```python
from build123d import *

# Parameters (mm, degrees)
SKETCH1_R           = 25
SKETCH1_R_2         = 5.1
SKETCH1_R_3         = 2.5
SKETCH1_W           = 36
SKETCH1_H           = 36
SKETCH1_W_2         = 6
SKETCH1_H_2         = 20
BOSS_EXTRUDE1_DEPTH = 3
BOSS_EXTRUDE2_DEPTH = 43
SKETCH4_W           = 11
SKETCH4_H           = 11
SKETCH4_W_2         = 7
SKETCH4_H_2         = 7
BOSS_EXTRUDE3_DEPTH = 5
SKETCH5_R           = 1.75
CUT_EXTRUDE1_DEPTH  = 5
SKETCH6_R           = 3.5
CUT_EXTRUDE2_DEPTH  = 3


with BuildPart() as part:
    # Sketch1 → Boss-Extrude1 (new body)
    with BuildSketch(Plane(origin=(0, 0, 0), x_dir=(1, 0, 0), z_dir=(0, 1, 0))):
        with BuildLine():
            Line((-20.833630945, -24.478740106), (119.166369055, -24.478740106))
            ThreePointArc((119.166369055, -24.478740106), (122.701902961, -23.014274012), (124.166369055, -19.478740106))
            Line((124.166369055, -19.478740106), (124.166369055, 72.136095087))
            ThreePointArc((124.166369055, 72.136095087), (123.306705208, 74.939239133), (121.023322437, 76.778478541))
            Line((121.023322437, 76.778478541), (75.060410419, 95.163643348))
            ThreePointArc((75.060410419, 95.163643348), (74.148994643, 95.431041828), (73.203457037, 95.521259894))
            Line((73.203457037, 95.521259894), (25.129281073, 95.521259894))
            ThreePointArc((25.129281073, 95.521259894), (24.183743467, 95.431041828), (23.272327691, 95.163643348))
            Line((23.272327691, 95.163643348), (-22.690584327, 76.778478541))
            ThreePointArc((-22.690584327, 76.778478541), (-24.973967097, 74.939239133), (-25.833630945, 72.136095087))
            Line((-25.833630945, 72.136095087), (-25.833630945, -19.478740106))
            ThreePointArc((-25.833630945, -19.478740106), (-24.369164851, -23.014274012), (-20.833630945, -24.478740106))
        make_face()
        with Locations((4.016369055, 8.771259894)):
            Circle(SKETCH1_R, mode=Mode.SUBTRACT)
        with Locations((94.316369055, 8.771259894)):
            Circle(SKETCH1_R, mode=Mode.SUBTRACT)
        with Locations((4.016369055, 67.521259894)):
            Circle(SKETCH1_R_2, mode=Mode.SUBTRACT)
        with Locations((94.316369055, 67.521259894)):
            Circle(SKETCH1_R_2, mode=Mode.SUBTRACT)
        with Locations((19.166369055, 79.316074422)):
            Circle(SKETCH1_R_3, mode=Mode.SUBTRACT)
        with Locations((19.166369055, 59.316074422)):
            Circle(SKETCH1_R_3, mode=Mode.SUBTRACT)
        with Locations((79.166369055, 59.316074422)):
            Circle(SKETCH1_R_3, mode=Mode.SUBTRACT)
        with Locations((79.166369055, 79.316074422)):
            Circle(SKETCH1_R_3, mode=Mode.SUBTRACT)
        with Locations((49.166369055, 67.521259894)):
            Rectangle(SKETCH1_W, SKETCH1_H, mode=Mode.SUBTRACT)
        with Locations((49.166369055, 8.771259894)):
            Rectangle(SKETCH1_W_2, SKETCH1_H_2, mode=Mode.SUBTRACT)
    extrude(amount=BOSS_EXTRUDE1_DEPTH)

    # Sketch2 → Boss-Extrude2 (add)
    with BuildSketch(Plane.XZ):
        with BuildLine():
            Line((-25.833630945, 19.478740106), (-25.833630945, -72.136095087))
            ThreePointArc((-25.833630945, -72.136095087), (-24.973967097, -74.939239133), (-22.690584327, -76.778478541))
            Line((-22.690584327, -76.778478541), (23.272327691, -95.163643348))
            ThreePointArc((23.272327691, -95.163643348), (24.183743467, -95.431041828), (25.129281073, -95.521259894))
            Line((25.129281073, -95.521259894), (73.203457037, -95.521259894))
            ThreePointArc((73.203457037, -95.521259894), (74.148994643, -95.431041828), (75.060410419, -95.163643348))
            Line((75.060410419, -95.163643348), (121.023322437, -76.778478541))
            ThreePointArc((121.023322437, -76.778478541), (123.306705208, -74.939239133), (124.166369055, -72.136095087))
            Line((124.166369055, -72.136095087), (124.166369055, 19.478740106))
            ThreePointArc((124.166369055, 19.478740106), (122.701902961, 23.014274012), (119.166369055, 24.478740106))
            Line((119.166369055, 24.478740106), (-20.833630945, 24.478740106))
            ThreePointArc((-20.833630945, 24.478740106), (-24.369164851, 23.014274012), (-25.833630945, 19.478740106))
        make_face()
        with BuildLine():
            Line((119.166369055, 21.478740106), (-20.833630945, 21.478740106))
            ThreePointArc((-20.833630945, 21.478740106), (-22.247844507, 20.892953668), (-22.833630945, 19.478740106))
            Line((-22.833630945, 19.478740106), (-22.833630945, -72.136095087))
            ThreePointArc((-22.833630945, -72.136095087), (-22.489765406, -73.257352705), (-21.576412297, -73.993048469))
            Line((-21.576412297, -73.993048469), (24.38649972, -92.378213276))
            ThreePointArc((24.38649972, -92.378213276), (24.751066031, -92.485172667), (25.129281073, -92.521259894))
            Line((25.129281073, -92.521259894), (73.203457037, -92.521259894))
            ThreePointArc((73.203457037, -92.521259894), (73.58167208, -92.485172667), (73.94623839, -92.378213276))
            Line((73.94623839, -92.378213276), (119.909150408, -73.993048469))
            ThreePointArc((119.909150408, -73.993048469), (120.822503516, -73.257352705), (121.166369055, -72.136095087))
            Line((121.166369055, -72.136095087), (121.166369055, 19.478740106))
            ThreePointArc((121.166369055, 19.478740106), (120.580582618, 20.892953668), (119.166369055, 21.478740106))
        make_face(mode=Mode.SUBTRACT)
    extrude(amount=BOSS_EXTRUDE2_DEPTH)

    # Sketch4 → Boss-Extrude3 (add)
    with BuildSketch(Plane.XZ):
        with Locations((79.166369055, -79.316074422)):
            Rectangle(SKETCH4_W, SKETCH4_H)
        with Locations((79.166369055, -79.316074422)):
            Rectangle(SKETCH4_W_2, SKETCH4_H_2, mode=Mode.SUBTRACT)
        with Locations((79.166369055, -59.316074422)):
            Rectangle(SKETCH4_W, SKETCH4_H)
        with Locations((79.166369055, -59.316074422)):
            Rectangle(SKETCH4_W_2, SKETCH4_H_2, mode=Mode.SUBTRACT)
        with Locations((19.166369055, -59.316074422)):
            Rectangle(SKETCH4_W, SKETCH4_H)
        with Locations((19.166369055, -59.316074422)):
            Rectangle(SKETCH4_W_2, SKETCH4_H_2, mode=Mode.SUBTRACT)
        with Locations((19.166369055, -79.316074422)):
            Rectangle(SKETCH4_W, SKETCH4_H)
        with Locations((19.166369055, -79.316074422)):
            Rectangle(SKETCH4_W_2, SKETCH4_H_2, mode=Mode.SUBTRACT)
    extrude(amount=BOSS_EXTRUDE3_DEPTH)

    # Sketch5 → Cut-Extrude1 (cut)
    with BuildSketch(Plane.XZ):
        with Locations((-17.833630945, 16.478740106)):
            Circle(SKETCH5_R)
        with Locations((116.166369055, 16.478740106)):
            Circle(SKETCH5_R)
        with Locations((-17.833630945, -63.521259894)):
            Circle(SKETCH5_R)
        with Locations((116.166369055, -63.521259894)):
            Circle(SKETCH5_R)
    extrude(amount=-CUT_EXTRUDE1_DEPTH, mode=Mode.SUBTRACT)

    # Sketch6 → Cut-Extrude2 (cut)
    with BuildSketch(Plane(origin=(0, 0, -95.521259894), x_dir=(-1, 0, 0), z_dir=(0, 0, -1))):
        with Locations((-49.166369055, -29.5)):
            Circle(SKETCH6_R)
    extrude(amount=-CUT_EXTRUDE2_DEPTH, mode=Mode.SUBTRACT)


solid = part.part
```
Check sheet for the modelled part. Datum: model origin and axes. Units: mm. A direction names the side the tool comes from. Coordinates: 2 decimals unless noted, no trailing zeros. Order: outer loops, then holes, each group sorted by start corner. A loop starts at its lowest first (then second) coordinate and runs counter-clockwise, first axis right, second up. Notation, with made-up numbers: M 70.5,46 L 99.5,46 A21 ccw 99.5,82 Z; hole C -36,5.5 d7. An arc over 180 degrees is marked long. One line per question, with ' | ' between items. Start each with the question number.
Item 1: Sectioned sample at C-C on y = -29.5. Record the cut outline in (x, z), and give its area (3 significant figures).
Item 2: Access from +Z, -Z, +X, -X, +Y, -Y to the whole of each face (thin tool, end or side, straight path). Record for faces 4 (the flat face through (22.666, -2, -59)), 5 (the flat face through (49, 1, -18.771)).
Item 3: Sectioned sample at B-B on z = 12.5. Record the cut outline in (x, y).
Item 4: Material ranges on line 1 (X direction, y = -21.5, z = 16); line 2 (Z direction, x = 74.5, y = -4); line 3 (Z direction, x = 40, y = -18), recorded low to high.
Item 5: Sectioned sample at D-D on x = 5. Record the cut outline in (y, z), and give its area (3 significant figures).
Item 6: Sectioned sample at A-A on x = 40. Record the cut outline in (y, z).
Item 7: Gauge pin test, flat ends, axial feed: P1, Ø12, axis at x = 51.5, z = -40.5, coming from the -Y side; P2, Ø3, axis at x = -17.83, z = 16.48, coming from the -Y side; P3, Ø4, axis at x = 31.5, z = -60.5, coming from the +Y side; P4, Ø1.5, axis at x = 17, y = -2, coming from the -Z side. Record the tip position at first contact, or that the pin passes through.
Item 8: Mould release check, pull along X, two halves, no side actions. Record for faces 1 (the flat face through (97.72, -19.68, -86.1)), 2 (the cylindrical face through (90.27, 1.48, -64.42)), 3 (the cylindrical face through (-24.33, -19.678, 23.053)): pulls with the +X half, pulls with the -X half, needs draft (parallel to the pull), parting line crosses it, or undercut.
Answer below:
1) outline: M -25.83,-72.14 A5 ccw -22.69,-76.78 L 23.27,-95.16 A5 ccw 25.13,-95.52 L 45.67,-95.52 L 45.67,-92.52 L 25.13,-92.52 A2 cw 24.39,-92.38 L -21.58,-73.99 A2 cw -22.83,-72.14 L -22.83,19.48 A2 cw -20.83,21.48 L 119.17,21.48 A2 cw 121.17,19.48 L 121.17,-72.14 A2 cw 119.91,-73.99 L 73.95,-92.38 A2 cw 73.2,-92.52 L 52.67,-92.52 L 52.67,-95.52 L 73.2,-95.52 A5 ccw 75.06,-95.16 L 121.02,-76.78 A5 ccw 124.17,-72.14 L 124.17,19.48 A5 ccw 119.17,24.48 L -20.83,24.48 A5 ccw -25.83,19.48 Z | area: 1,460 mm^2
2) face 4: -Y | face 5: +Y, -Y
3) outline: M -25.83,-43 L -22.83,-43 L -22.83,0 L -9.12,0 L -9.12,3 L -25.83,3 Z; M 17.15,0 L 81.18,0 L 81.18,3 L 17.15,3 Z; M 107.45,0 L 121.17,0 L 121.17,-43 L 124.17,-43 L 124.17,3 L 107.45,3 Z
4) line 1: x = -25.83 to -22.83, 121.17 to 124.17 | line 2: z = -95.35 to -92.16, -84.82 to -73.82, -64.82 to -53.82, 21.48 to 24.48 | line 3: z = -95.52 to -92.52, 21.48 to 24.48
5) outline: M -43,-87.85 L 3,-87.85 L 3,-72.53 L 0,-72.53 L 0,-84.62 L -43,-84.62 Z; M -43,21.48 L 0,21.48 L 0,16.21 L 3,16.21 L 3,24.48 L -43,24.48 Z; M 0,-62.52 L 3,-62.52 L 3,-33.75 L 0,-33.75 Z | area: 425 mm^2
6) outline: M -43,-95.52 L 3,-95.52 L 3,-85.52 L 0,-85.52 L 0,-92.52 L -43,-92.52 Z; M -43,21.48 L 0,21.48 L 0,-49.52 L 3,-49.52 L 3,24.48 L -43,24.48 Z
7) P1: stops at y = 0 | P2: passes through | P3: stops at y = 3 | P4: stops at z = -92.95
8) face 1: pulls with the +X half | face 2: undercut | face 3: pulls with the -X half
